Design review of the part built by this model. Coordinates are the model's own, in mm. Face numbers are marked on the shaded views. A direction names the side the tool comes from. Coordinates: 2 decimals unless noted, no trailing zeros. Order: outer loops, then holes, each group sorted by start corner. A loop starts at its lowest first (then second) coordinate and runs counter-clockwise, first axis right, second up.
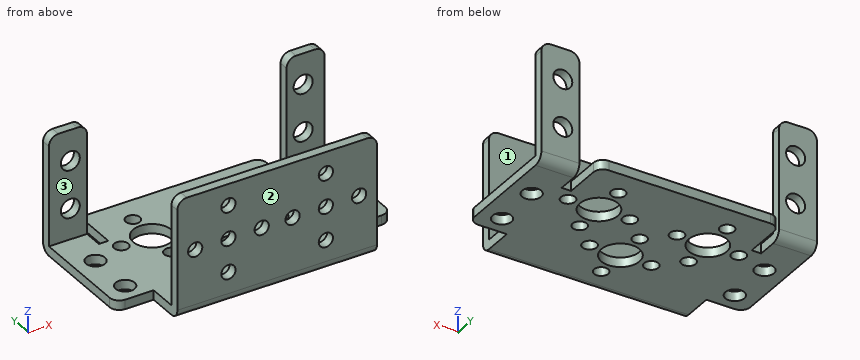
from build123d import *

# Parameters (mm, degrees)
PAD_DEPTH       = 2
SKETCH001_W     = 8
SKETCH001_H     = 2
SKETCH001_W_2   = 42
PAD001_DEPTH    = 23
SKETCH002_R     = 1.5
SKETCH002_R_2   = 4
SKETCH002_R_3   = 2
POCKET_DEPTH    = 5
SKETCH003_R     = 2
SKETCH003_R_2   = 1.5
POCKET001_DEPTH = 32.501
FILLET_R        = 2
FILLET001_R     = 1.99


with BuildPart() as part:
    # Sketch → Pad (new body)
    with BuildSketch(Plane.XY):
        with BuildLine():
            Line((0, -18), (21, -18))
            Line((21, -18), (21, -10))
            Line((21, -10), (27, -10))
            ThreePointArc((27, -10), (28.414214, -9.414214), (29, -8))
            Line((29, -8), (29, 14.5))
            Line((29, 14.5), (21, 14.5))
            Line((21, 14.5), (21, 8.5))
            Line((21, 8.5), (19, 8.5))
            Line((19, 8.5), (19, 16))
            ThreePointArc((19, 16), (18.414214, 17.414214), (17, 18))
            Line((17, 18), (0, 18))
            Line((0, 18), (0, -18))
        make_face()
    pad = extrude(amount=PAD_DEPTH)

    # Mirrored: Pad across Sketch V_Axis
    add(pad.mirror(Plane(origin=(0, 0, 0), x_dir=(0, 0, 1), z_dir=(1, 0, 0))))

    # Sketch001 (on Face5 of Mirrored) → Pad001 (join)
    with BuildSketch(Plane.XY.offset(2)):
        with Locations((25, 13.5)):
            Rectangle(SKETCH001_W, SKETCH001_H)
        with Locations((-25, 13.5)):
            Rectangle(SKETCH001_W, SKETCH001_H)
        with Locations((0, -17)):
            Rectangle(SKETCH001_W_2, SKETCH001_H)
    extrude(amount=PAD001_DEPTH)

    # Sketch002 (on Face10 of Pad001) → Pocket (cut)
    with BuildSketch(Plane.XY.offset(2)):
        with Locations((-11.46, 12.3)):
            Circle(SKETCH002_R)
        with Locations((-11.46, 5.8)):
            Circle(SKETCH002_R_2)
        with Locations((-4.96, 5.8)):
            Circle(SKETCH002_R)
        with Locations((-17.96, 5.8)):
            Circle(SKETCH002_R)
        with Locations((-11.46, -0.7)):
            Circle(SKETCH002_R)
        with Locations((11.46, 12.3)):
            Circle(SKETCH002_R)
        with Locations((11.46, 5.8)):
            Circle(SKETCH002_R_2)
        with Locations((4.96, 5.8)):
            Circle(SKETCH002_R)
        with Locations((17.96, 5.8)):
            Circle(SKETCH002_R)
        with Locations((11.46, -0.7)):
            Circle(SKETCH002_R)
        with Locations((0, 1.171128)):
            Circle(SKETCH002_R)
        with Locations((0, -5.328872)):
            Circle(SKETCH002_R_2)
        with Locations((6.5, -5.328872)):
            Circle(SKETCH002_R)
        with Locations((-6.5, -5.328872)):
            Circle(SKETCH002_R)
        with Locations((0, -11.828872)):
            Circle(SKETCH002_R)
        with Locations((-24.5, 4)):
            Circle(SKETCH002_R_3)
        with Locations((-24.5, -6)):
            Circle(SKETCH002_R_3)
        with Locations((24.5, 4)):
            Circle(SKETCH002_R_3)
        with Locations((24.5, -6)):
            Circle(SKETCH002_R_3)
    extrude(amount=-POCKET_DEPTH, mode=Mode.SUBTRACT)

    # Sketch003 (on Face53 of Pocket) → Pocket001 (cut, through all)
    with BuildSketch(Plane(origin=(0, 14.5, 0), x_dir=(-1, 0, 0), z_dir=(0, 1, 0))):
        with Locations((-24.5, 18.5)):
            Circle(SKETCH003_R)
        with Locations((-24.5, 8.5)):
            Circle(SKETCH003_R)
        with Locations((24.5, 18.5)):
            Circle(SKETCH003_R)
        with Locations((24.5, 8.5)):
            Circle(SKETCH003_R)
        with Locations((-10.25, 20.5)):
            Circle(SKETCH003_R_2)
        with Locations((-10.25, 13.5)):
            Circle(SKETCH003_R_2)
        with Locations((-10.25, 6.5)):
            Circle(SKETCH003_R_2)
        with Locations((-3.25, 13.5)):
            Circle(SKETCH003_R_2)
        with Locations((-17.25, 13.5)):
            Circle(SKETCH003_R_2)
        with Locations((10.25, 20.5)):
            Circle(SKETCH003_R_2)
        with Locations((10.25, 13.5)):
            Circle(SKETCH003_R_2)
        with Locations((10.25, 6.5)):
            Circle(SKETCH003_R_2)
        with Locations((3.25, 13.5)):
            Circle(SKETCH003_R_2)
        with Locations((17.25, 13.5)):
            Circle(SKETCH003_R_2)
    extrude(amount=-POCKET001_DEPTH, mode=Mode.SUBTRACT)

    # Fillet
    fillet_edges = [part.edges().sort_by_distance(p)[0] for p in [
        (29, 13.5, 25),
        (21, 13.5, 25),
        (21, -17, 25),
        (-21, -17, 25),
        (-21, 13.5, 25),
        (-29, 13.5, 25),
    ]]
    fillet(fillet_edges, radius=FILLET_R)

    # Fillet001
    fillet001_edges = [part.edges().sort_by_distance(p)[0] for p in [
        (25, 14.5, 0),
        (-25, 14.5, 0),
        (-10.5, -18, 0),
        (10.5, -18, 0),
    ]]
    fillet(fillet001_edges, radius=FILLET001_R)


solid = part.part
1. Add section D-D (y = 5). State how many separate pieces and enclosed holes the cut face has, and give its area (3 significant figures).
2. To check wall thickness, follow line 1 (Y direction, x = 11.46, z = 0.4); line 2 (Z direction, x = 24.5, y = 14.05); line 3 (Y direction, x = 24.5, z = 0.65). State the ranges of each line that lie inside material, in increasing order.
3. Add section C-C (y = -14). Give the boundary of the cut face in (x, z).
4. For the marked faces 1, 2 and 3, list the 3-axis set-ups (+Z, -Z, +X, -X, +Y, -Y) from which the entire face can be reached by the end or side of a thin tool; tool diameter is ignored.
5. Add section A-A (z = 3). Give the boundary of the cut face in (x, y).
6. Add section B-B (x = 24.5). Give the boundary of the cut face in (y, z), and give its area (4 significant figures).
7. Insertion check: pin 1 (10 mm diameter, centred on x = -13.5, y = -6.5, fed in from +Z); pin 2 (1.8 mm diameter, centred on x = 11.46, y = 12.3, fed in from +Z); pin 3 (0.6 mm diameter, centred on x = 24, z = 1, fed in from -Y); pin 4 (6.5 mm diameter, centred on x = 23.5, z = 17.5, fed in from +Y). Each pin has a flat end and moves straight along its axis. Give the tip position at first contact, or say it passes through.
Solution:
1. separate pieces: 9
1. enclosed holes: 0
1. area: 50.5 mm2
2. line 1: y = -17.21 to -2.2, 0.8 to 1.8, 9.8 to 10.8, 13.8 to 18
2. line 2: z = 0.73 to 6.5, 10.5 to 16.5, 20.5 to 25
2. line 3: y = -10 to -8, -4 to 2, 6 to 13.98
3. outline: (-21, 0) - (21, 0) - (21, 2) - (-21, 2) - close
4. face 1: +Z, +X, -X, +Y
4. face 2: +Z, -Z, +X, -X, -Y
4. face 3: +Z, +X, -X, -Y
5. outline: (-29, 12.5) - (-21, 12.5) - (-21, 14.5) - (-29, 14.5) - close; (-21, -18) - (21, -18) - (21, -16) - (-21, -16) - close; (21, 12.5) - (29, 12.5) - (29, 14.5) - (21, 14.5) - close
6. outline: (-10, 0) - (-8, 0) - (-8, 2) - (-10, 2) - close; (-4, 0) - (2, 0) - (2, 2) - (-4, 2) - close; (6, 0) - (12.51, 0) arc R1.99 ccw to (14.5, 1.99) - (14.5, 6.5) - (12.5, 6.5) - (12.5, 2) - (6, 2) - close; (12.5, 10.5) - (14.5, 10.5) - (14.5, 16.5) - (12.5, 16.5) - close; (12.5, 20.5) - (14.5, 20.5) - (14.5, 25) - (12.5, 25) - close
6. area: 62.15 mm2
7. pin 1: stops at z = 2
7. pin 2: passes through
7. pin 3: stops at y = -10
7. pin 4: stops at y = 14.5
